Can you work these out from the model? Positions are in its coordinate system, mm. A direction names the side the tool comes from. Round coordinates to 2 decimals unless told otherwise and drop trailing zeros. Order: outer loops, then holes, each group sorted by start corner. A loop starts at its lowest first (then second) coordinate and runs counter-clockwise, first axis right, second up. Notation, with made-up numbers: M -1.5,44.5 L 23.5,44.5 A21 ccw 23.5,70.5 Z; hole C 60.5,12 d8. An arc over 180 degrees is marked long. Answer as a JSON object with one key per item and string values. Group by question number.
from build123d import *

# Parameters (mm, degrees)
SKETCH_1_W          = 47
SKETCH_1_H          = 17
SKETCH_1_W_2        = 42
SKETCH_1_H_2        = 11
EXTRUDE_1_DEPTH     = 10
SKETCH_2_W          = 47
SKETCH_2_H          = 17
EXTRUDE_2_DEPTH     = 3
SKETCH_3_W          = 6
SKETCH_3_H          = 11
CUT_EXTRUDE_2_DEPTH = 3


with BuildPart() as part:
    # 草圖1 → 填料-伸長1 (new body)
    with BuildSketch(Plane.XY):
        with Locations((8.49357684, 1.797560976)):
            Rectangle(SKETCH_1_W, SKETCH_1_H)
        with Locations((8.49357684, 1.797560976)):
            Rectangle(SKETCH_1_W_2, SKETCH_1_H_2, mode=Mode.SUBTRACT)
    extrude(amount=EXTRUDE_1_DEPTH)

    # 草圖2 → 填料-伸長2 (add)
    with BuildSketch(Plane(origin=(0, 0, 0), x_dir=(-1, 0, 0), z_dir=(0, 0, -1))):
        with Locations((-8.49357684, 1.797560976)):
            Rectangle(SKETCH_2_W, SKETCH_2_H)
    extrude(amount=EXTRUDE_2_DEPTH)

    # 草圖3 → 除料-伸長2 (cut)
    with BuildSketch(Plane(origin=(31.99357684, 0, 0), x_dir=(0, 0, -1), z_dir=(1, 0, 0))):
        with Locations((-7, 1.797560976)):
            Rectangle(SKETCH_3_W, SKETCH_3_H)
    extrude(amount=-CUT_EXTRUDE_2_DEPTH, mode=Mode.SUBTRACT)


solid = part.part
Item 1: I'm going to push flat-ended pins straight in: pin 1 Ø3 at (x, y) = (-9.5, -1.5) entering from +Z; pin 2 Ø3 at (x, y) = (30.5, 4) entering from +Z. Where does each tip first touch, or does it pass through?
Item 2: Suppose I cut it at C-C, the plane y = -2.25. Write out the boundary of the cut face in (x, z), and give its area (3 significant figures).
Item 3: I need wall thicknesses on line 1 (Y direction, x = 7, z = 2.5); line 2 (X direction, y = 4, z = 1.5); line 3 (Z direction, x = 20, y = 2.25). Which ranges of each line are inside material? Lowest first, please.
Item 4: Suppose I cut it at B-B, the plane x = -7. Write out the boundary of the cut face in (y, z), and give its area (3 significant figures).
Item 5: If we mould it in two halves opening along X, with no side actions, what happens to faces 1 (the face through (29.494, 2, 2)), 2 (the face through (31.994, 2, 2)), 3 (the face through (8, 8, 10)), 4 (the face through (-15.006, 2, 4))? For each: +X half, -X half, draft (parallel to the pull), parting line (faces both ways), or undercut.
Item 6: Suppose I cut it at A-A, the plane z = 1. Write out the boundary of the cut face in (x, y).
Item 7: On a 3-axis mill with a long thin cutter (end or side, diameter ignored), from which of +Z, -Z, +X, -X, +Y, -Y can I reach the whole of each face in a straight line? I mean faces 5 (the face through (9, 10.298, 4)), 6 (the face through (-12.506, 2, 5)), 7 (the face through (31, 2, 4)). Say none if no direction works.
Computed:
{
 "1": {"pin 1": "stops at z = 0", "pin 2": "stops at z = 4"},
 "2": {"outline": "M -15.01,-3 L 31.99,-3 L 31.99,4 L 29.49,4 L 29.49,0 L -12.51,0 L -12.51,10 L -15.01,10 Z", "area": "176 mm^2"},
 "3": {"line 1": "y = -6.7 to -3.7, 7.3 to 10.3", "line 2": "x = -15.01 to -12.51, 29.49 to 31.99", "line 3": "z = -3 to 0"},
 "4": {"outline": "M -6.7,-3 L 10.3,-3 L 10.3,10 L 7.3,10 L 7.3,0 L -3.7,0 L -3.7,10 L -6.7,10 Z", "area": "111 mm^2"},
 "5": {"face 1": "undercut", "face 2": "+X half", "face 3": "draft", "face 4": "-X half"},
 "6": {"outline": "M -15.01,-6.7 L 31.99,-6.7 L 31.99,10.3 L -15.01,10.3 Z; hole M -12.51,-3.7 L 29.49,-3.7 L 29.49,7.3 L -12.51,7.3 Z"},
 "7": {"face 5": "+Z, -Z, +X, -X, +Y", "face 6": "+Z", "face 7": "+Z, +X"}
}
